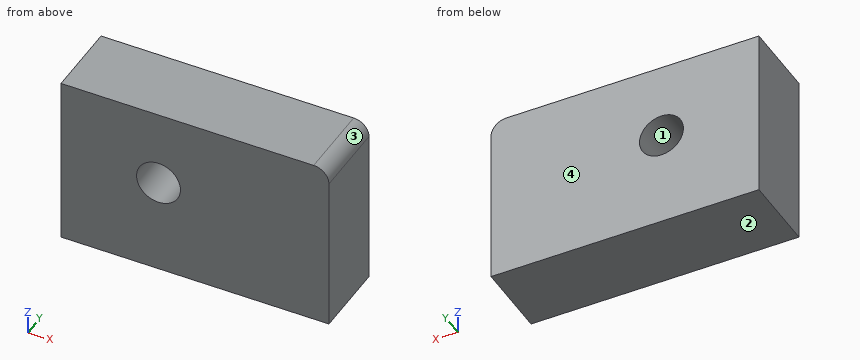
from build123d import *

# Parameters (mm, degrees)
F0_W     = 88.971116
F0_H     = 57.607204
F1_DEPTH = 12.7
F2_R     = 7.295554
F3_DEPTH = 25.4
F4_R     = 5.08


with BuildPart() as f1:
    # F0 (on Front) → F1 (new body, symmetric)
    with BuildSketch(Plane.XZ):
        Rectangle(F0_W, F0_H)
    extrude(amount=F1_DEPTH, both=True)

    # F2 (on face) → F3 (cut, through all)
    with BuildSketch(Plane.XZ.offset(12.7)):
        with Locations((-12.114964, 3.403602)):
            Circle(F2_R)
    extrude(amount=-F3_DEPTH, mode=Mode.SUBTRACT)

    # F4
    f4_edges = [f1.edges().sort_by_distance(p)[0] for p in [
        (44.485558, 0, 28.803602),
    ]]
    fillet(f4_edges, radius=F4_R)


solid = f1.part
Here's how the part is built. I have some questions about the finished solid (model axes, mm). Face numbers are marked on the shaded views. Round coordinates to 2 decimals unless told otherwise and drop trailing zeros. Write each loop counter-clockwise with the first axis right and the second up, starting at its lowest first coordinate (ties: lowest second). Pieces come first, ordered by that corner, then holes.
1. If we mould it in two halves opening along Z, with no side actions, what happens to the marked faces 1, 2, 3 and 4? For each: released by +Z, released by -Z, zero draft, split by the parting line, or undercut.
2. Will this pin go through, and if not, where does the flat tip stop? pin 1 Ø13 at (x, z) = (-12.11, 3.4) entering from -Y.
3. Suppose I cut it at A-A (x = -9). List the corners of the cut face in (y, z) for me.
4. Suppose I cut it at B-B (z = 2.5). List the corners of the cut face in (x, y) for me.
5. Suppose I cut it at C-C (y = 1). List the corners of the cut face in (x, z) for me, and give its area (3 significant figures).
6. I need wall thicknesses on L1, parallel to X at y = -0.75, z = 2; L2, parallel to X at y = 1.25, z = 6. Which ranges of each line are inside material? Lowest first, please.
Answer sheet:
1. face 1: undercut
1. face 2: released by -Z
1. face 3: released by +Z
1. face 4: zero draft
2. pin 1: passes through
3. outline: (-12.7, -28.8) - (12.7, -28.8) - (12.7, -3.19) - (-12.7, -3.19) - close; (-12.7, 10) - (12.7, 10) - (12.7, 28.8) - (-12.7, 28.8) - close
4. outline: (-44.49, -12.7) - (-19.35, -12.7) - (-19.35, 12.7) - (-44.49, 12.7) - close; (-4.88, -12.7) - (44.49, -12.7) - (44.49, 12.7) - (-4.88, 12.7) - close
5. outline: (-44.49, -28.8) - (44.49, -28.8) - (44.49, 23.72) arc R5.08 ccw to (39.41, 28.8) - (-44.49, 28.8) - close; hole circle Ø14.59 at (-12.11, 3.4)
5. area: 4,950 mm2
6. L1: x = -44.49 to -19.27, -4.96 to 44.49
6. L2: x = -44.49 to -18.93, -5.3 to 44.49
